Verification items for the finished model (mm, model axes). Face numbers are marked on the shaded views. A direction names the side the tool comes from. Give positions to 0.01 mm unless a question says otherwise; leave off trailing zeros. Write each loop counter-clockwise with the first axis right and the second up, starting at its lowest first coordinate (ties: lowest second). Pieces come first, ordered by that corner, then holes. Notation, with made-up numbers: (-13.75, 5.5) - (33.25, 5.5) arc R27 ccw to (33.25, 36.5) - close; hole circle Ø1 at (85.25, -4). An arc over 180 degrees is marked (long way). Answer as a JSON object with one key per item and string values. Group by question number.
Item 1: Tool access check on the marked faces 4 and 5. Record the directions out of +Z, -Z, +X, -X, +Y, -Y that give a thin tool (end or side, any length) a straight path to the whole face; none if there is none.
Item 2: Scan lines: line 1 along Y through (x, z) = (43.5, -7); line 2 along Y through (x, z) = (34, -1.25); line 3 along Y through (x, z) = (7, -7.5). Record each from-to range of solid material in increasing order. Write a range as [from, to].
Item 3: Go/stop test with flat-tipped pins: pin 1 (3 mm diameter, centred on y = -32.5, z = -7, fed in from -X); pin 2 (3 mm diameter, centred on x = 27.5, z = -6, fed in from -Y); pin 3 (5 mm diameter, centred on y = -23.5, z = -7.5, fed in from -X). Record where each tip stops, or that it passes through.
Item 4: Draft check along Y on the marked faces 1, 2 and 3. Enter one of: +Y half, -Y half, draft (parallel to the pull), parting line (faces both ways), or undercut.
Item 5: Sectioned sample at A-A, the plane x = 38. Record the boundary of the cut face in (y, z), and give its area (3 significant figures).
Item 6: Sectioned sample at B-B, the plane y = -39. Record the boundary of the cut face in (x, z).
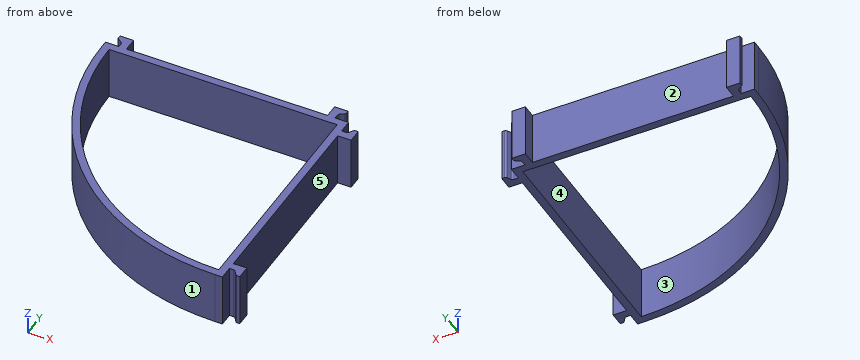
Autodesk Inventor part; units mm, degrees
ref_plane "YZ Plane" through (0, 0, 0) normal (1, 0, 0) x (0, 1, 0)
ref_plane "XZ Plane" through (0, 0, 0) normal (0, 1, 0) x (-1, 0, 0)
ref_plane "XY Plane" through (0, 0, 0) normal (0, 0, 1) x (1, 0, 0)
sketch "Boceto1" plane through (0, 0, 0) normal (0, 0, 1) x (1, 0, 0)
  line L0 (43.6, -1.4) -> (1.4, -1.4)
  line L1 (0, -1.4) -> (0, 0)
  line L2 (45, -45) -> (43.6, -45)
  line L3 (43.6, -43.6) -> (43.6, -1.4)
  arc A0 (1.4, -1.4) -> (43.6, -43.6) centre (43.6, -1.4) ccw
  arc A1 (0, -1.4) -> (43.6, -45) centre (43.6, -1.4) ccw
  line L4 (2.5, 0) -> (2.5, 0.7532)
  line L5 (2.2918, 1.1592) -> (1.4, 1.8)
  line L6 (1.4, 1.8) -> (1.4, 2.5)
  line L7 (1.4, 2.5) -> (3.9, 2.5)
  line L8 (3.9, 2.5) -> (3.9, 0)
  arc A2 (2.5, 0.7532) -> (2.2918, 1.1592) centre (2, 0.7532) ccw
  line L9 (0, 0) -> (2.5, 0)
  line L10 (42.5, 0) -> (42.5, 0.8223)
  line L11 (42.7447, 1.2522) -> (43.3553, 1.6147)
  line L12 (43.6, 2.0446) -> (43.6, 2.5)
  line L13 (43.6, 2.5) -> (41.1, 2.5)
  line L14 (41.1, 2.5) -> (41.1, 0)
  line L15 (3.9, 0) -> (41.1, 0)
  line L16 (42.5, 0) -> (45, 0)
  arc A3 (42.7447, 1.2522) -> (42.5, 0.8223) centre (43, 0.8223) ccw
  arc A4 (43.3553, 1.6147) -> (43.6, 2.0446) centre (43.1, 2.0446) ccw
  line L17 (45, -2.5) -> (45.8223, -2.5)
  line L18 (46.2522, -2.2553) -> (46.6147, -1.6447)
  line L19 (47.0446, -1.4) -> (47.5, -1.4)
  line L20 (47.5, -1.4) -> (47.5, -3.9)
  line L21 (47.5, -3.9) -> (45, -3.9)
  arc A5 (47.0446, -1.4) -> (46.6147, -1.6447) centre (47.0446, -1.9) ccw
  arc A6 (45.8223, -2.5) -> (46.2522, -2.2553) centre (45.8223, -2) ccw
  line L22 (45, -42.5) -> (45.7532, -42.5)
  line L23 (46.1592, -42.7082) -> (46.8, -43.6)
  line L24 (46.8, -43.6) -> (47.5, -43.6)
  line L25 (47.5, -43.6) -> (47.5, -41.1)
  line L26 (47.5, -41.1) -> (45, -41.1)
  arc A7 (46.1592, -42.7082) -> (45.7532, -42.5) centre (45.7532, -43) ccw
  line L27 (45, -0.1052) -> (45, -2.5)
  line L28 (45, -2.5) -> (45, 0)
  line L29 (45, -3.9) -> (45, -41.1)
  line L30 (45, -42.5) -> (45, -45)
  line L31 (45, -45) -> (45, -42.5)
  line L32 (45, -41.1) -> (45, -3.9)
  point P0 (43.6, 1.76)
  point P1 (46.76, -1.4)
  dimension "d11" = 42.2
  dimension "d12" = 1.4
  dimension "d18" = 1.4
  dimension "d19" = 2.5
  dimension "d21" = 2.5
  dimension "d25" = 35.7
  dimension "d26" = 1.4
  dimension "d28" = 1.4
  dimension "d29" = 0.74
  dimension "d30" = 2.5
  dimension "d31" = 30.7
  dimension "d32" = 2.5
  dimension "d34" = 0.5
  dimension "d35" = 0.7
  dimension "d36" = 0.5
  dimension "d37" = 0.5
  dimension "d38" = 1.4
  dimension "d39" = 2.5
  dimension "d41" = 2.5
  dimension "d42" = 0.74
  dimension "d43" = 30.7
  dimension "d44" = 0.5
  dimension "d45" = 45
  dimension "d46" = 1.4
  dimension "d47" = 2.5
  dimension "d49" = 0.7
  dimension "d50" = 35.7
  dimension "d51" = 2.5
  dimension "d52" = 0.5
  dimension "d55" = 1.4
  dimension "d57" = 2.5
  dimension "d58" = 45
  dimension "d59" = 2.5
  dimension "d63" = 2.5
  dimension "d64" = 2.5
extrude "Extrusión1" add sketch "Boceto1" against normal blind 10
properties part number "SP40-15 PERFIL ESQUINERO PUNTAS INVERTIDAS" material "Aluminio"
Geometry check:
{
 "1": {"face 4": "+Z, -Z", "face 5": "+Z, -Z, +X"},
 "2": {"line 1": "[-45, -43.6], [-1.4, 0], [1.74, 2.5]", "line 2": "[-43.93, -42.49], [-1.4, 0]", "line 3": "[-25.09, -22.41], [-1.4, 0]"},
 "3": {"pin 1": "x = 11.59", "pin 2": "y = -42.48", "pin 3": "x = 4.65"},
 "4": {"face 1": "-Y half", "face 2": "+Y half", "face 3": "undercut"},
 "5": {"outline": "(-44.64, -10) - (-43.23, -10) - (-43.23, 0) - (-44.64, 0) - close; (-1.4, -10) - (0, -10) - (0, 0) - (-1.4, 0) - close", "area": "28.1 mm^2"},
 "6": {"outline": "(21.53, -10) - (24.44, -10) - (24.44, 0) - (21.53, 0) - close; (43.6, -10) - (45, -10) - (45, 0) - (43.6, 0) - close"}
}
